The drawing under review shows one solid part. Ordinate dimensions are in mm from its lowest x, y, z. A direction names the side the tool comes from. Give positions to 0.01 mm unless a question says otherwise; leave off trailing zeros. Order: outer loops, then holes, each group sorted by start corner. A loop starts at its lowest first (then second) coordinate and runs counter-clockwise, first axis right, second up. Notation, with made-up numbers: (42.25, 15.5) -> (89.25, 15.5) arc R26 cw to (89.25, 33.5) -> close; hole circle Ø3 at (77, 20.5). An arc over 180 degrees is marked (long way). Return JSON: item names as keys, results as strings. Group by question number.
1) Add section C-C (x = 9). Give the boundary of the cut face in (y, z).
2) Add section B-B (z = 54). Give the boundary of the cut face in (x, y), then the cut area to 3 significant figures.
3) To check wall thickness, follow line 1 along Z through (x, y) = (12.5, 0.55); line 2 along Y through (x, z) = (6.25, 9); line 3 along Z through (x, y) = (18.25, 3.25). State the ranges of each line that lie inside material, in increasing order.
4) Add section A-A (x = 12.5). Give the boundary of the cut face in (y, z).
5) For the marked faces 1 and 2, list the 3-axis set-ups (+Z, -Z, +X, -X, +Y, -Y) from which the entire face can be reached by the end or side of a thin tool; tool diameter is ignored.
6) Insertion check: P1, Ø1.6, axis at x = 10.5, y = 3, coming from the +Z side; P2, Ø2, axis at y = 3.5, z = 49.5, coming from the -X side; P3, Ø1, axis at x = 20, z = 32, coming from the +Y side. Each pin has a flat end and moves straight along its axis. Give the tip position at first contact, or say it passes through.
7) Add section D-D (y = 3). Give the boundary of the cut face in (x, z), then the cut area to 3 significant figures.
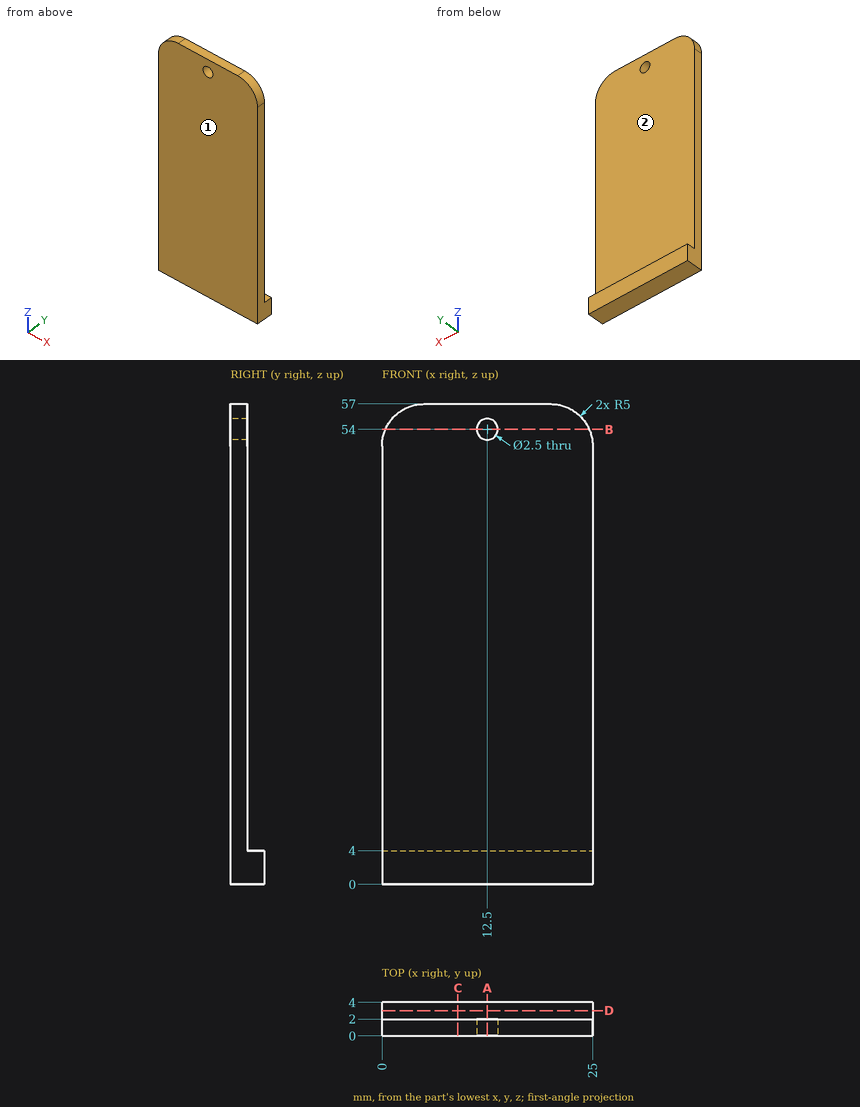
Evaluation:
{
 "1": {"outline": "(0, 0) -> (4, 0) -> (4, 4) -> (2, 4) -> (2, 57) -> (0, 57) -> close"},
 "2": {"outline": "(0.42, 0) -> (11.25, 0) -> (11.25, 2) -> (0.42, 2) -> close; (13.75, 0) -> (24.58, 0) -> (24.58, 2) -> (13.75, 2) -> close", "area": "43.3 mm^2"},
 "3": {"line 1": "0 to 52.75, 55.25 to 57", "line 2": "0 to 2", "line 3": "0 to 4"},
 "4": {"outline": "(0, 0) -> (4, 0) -> (4, 4) -> (2, 4) -> (2, 52.75) -> (0, 52.75) -> close; (0, 55.25) -> (2, 55.25) -> (2, 57) -> (0, 57) -> close"},
 "5": {"face 1": "+Z, -Z, +X, -X, -Y", "face 2": "+Z, +X, -X, +Y"},
 "6": {"P1": "z = 4", "P2": "through", "P3": "y = 2"},
 "7": {"outline": "(0, 0) -> (25, 0) -> (25, 4) -> (0, 4) -> close", "area": "100 mm^2"}
}
